The model under review builds one solid part; all positions refer to its coordinate system, in mm. A direction names the side the tool comes from. Round coordinates to 2 decimals unless told otherwise and drop trailing zeros. Write each loop counter-clockwise with the first axis right and the second up, starting at its lowest first coordinate (ties: lowest second). Pieces come first, ordered by that corner, then holes. Notation, with made-up numbers: (-12.75, -2.75) -> (33.25, -2.75) arc R24 ccw to (33.25, 16.25) -> close; hole circle Ø3 at (21.5, 21.25). An arc over 180 degrees is marked (long way). Answer as a JSON object with one key per item and string values. Group by question number.
1) To check wall thickness, follow probe 1 along X at (y, z) = (9.25, 15.75); probe 2 along Y at (x, z) = (-4.5, 16.25); probe 3 along Y at (x, z) = (-1, 19). State the ranges of each line that lie inside material, in increasing order. Write a range as [from, to].
2) We need section B-B, the plane y = 7. Write out the cut boundary in (x, z).
3) Machinability: for faces 4 (the flat face through (0, 6, -1.78)), 5 (the flat face through (-6.452, 5, 18)), 6 (the cylindrical face through (4.61, -1.38, 7.48)), 7 (the flat face through (-8.89, 5, 10)), 8 (the flat face through (8.39, -2, 9)), which of the approach directions +Z, -Z, +X, -X, +Y, -Y give a long, thin tool a straight path to every point of the face, cutting with its end or side? Answer none if there is none.
4) We need section A-A, the plane y = -0.5. Count the separate pieces of the cut face and the enclosed holes in it, then the cut area to 3 significant figures.
5) We need section D-D, the plane y = 10. Write out the cut boundary in (x, z).
6) Insertion check: pin 1 Ø6 at (x, z) = (-6.5, 20) entering from -Y; pin 2 Ø2 at (x, y) = (-1.5, 3) entering from +Z; pin 3 Ø2 at (x, z) = (3.5, 12.5) entering from -Y. Each pin has a flat end and moves straight along its axis. Give the tip position at first contact, or say it passes through.
7) Mouldability with a two-part tool opening along Z and no side actions: class faces 1 (the flat face through (0, 10.404, 18)), 2 (the cylindrical face through (-5.04, -1.38, 7.48)), 3 (the flat face through (-5, 10, 22.45)) as pulls with the +Z half, pulls with the -Z half, needs draft (parallel to the pull), parting line crosses it, or undercut.
8) We need section C-C, the plane z = 9.14. Write out the cut boundary in (x, y), then the cut area to 3 significant figures.
Autodesk Inventor part; units mm, degrees
ref_plane "YZ Plane" through (0, 0, 0) normal (1, 0, 0) x (0, 1, 0)
ref_plane "XZ Plane" through (0, 0, 0) normal (0, 1, 0) x (-1, 0, 0)
ref_plane "XY Plane" through (0, 0, 0) normal (0, 0, 1) x (1, 0, 0)
sketch "Sketch1" plane through (0, 0, 0) normal (0, 1, 0) x (-1, 0, 0)
  line L0 (8.89, 22.35) -> (-8.89, 22.35)
  line L1 (-8.89, 22.35) -> (-8.89, -1.78)
  line L2 (-8.89, -1.78) -> (8.89, -1.78)
  line L3 (8.89, -1.78) -> (8.89, 22.35)
  point P0 (0, 0)
  dimension "d0" = 24.13
  dimension "d1" = 22.35
  dimension "d2" = 17.78
  dimension "d3" = 8.89
extrude "Extrusion1" add sketch "Sketch1" along normal blind 11.25
sketch "Sketch2" plane through (-8.89, 0, 22.35) normal (0, 0, 1) x (1, 0, 0)
  line L0 (2.4376, 1.9143) -> (15.6231, 1.9143)
  line L1 (15.6231, 1.9143) -> (15.6231, 8.5296)
  line L2 (15.6231, 8.5296) -> (2.4376, 8.5296)
  line L3 (2.4376, 8.5296) -> (2.4376, 1.9143)
  line L4 (6.2307, 8.5296) -> (11.6268, 8.5296)
  line L5 (11.6268, 8.5296) -> (11.6268, 10.4036)
  line L6 (11.6268, 10.4036) -> (6.2307, 10.4036)
  line L7 (6.2307, 10.4036) -> (6.2307, 8.5296)
  point P0 (8.89, 0)
extrude "Extrusion2" cut sketch "Sketch2" against normal blind 8
sketch "Sketch3" plane through (-8.89, 0, 22.35) normal (0, 0, 1) x (1, 0, 0)
  line L0 (12.4503, 9.0228) -> (15.6135, 9.0228)
  line L1 (15.6135, 9.0228) -> (15.6135, 10.4036)
  line L2 (15.6135, 10.4036) -> (12.4503, 10.4036)
  line L3 (12.4503, 10.4036) -> (12.4503, 9.0228)
  line L4 (5.8403, 9.0228) -> (2.4376, 9.0228)
  line L5 (2.4376, 9.0228) -> (2.4376, 10.4036)
  line L6 (2.4376, 10.4036) -> (5.8403, 10.4036)
  line L7 (5.8403, 10.4036) -> (5.8403, 9.0228)
  point P0 (8.89, 0)
extrude "Extrusion3" add sketch "Sketch3" along normal blind 0.1
sketch "Sketch4" plane through (8.89, 0, 22.35) normal (1, 0, 0) x (0, 0, -1)
  line L0 (12.46, 3.4608) -> (13.96, 3.4608)
  line L1 (13.96, 3.4608) -> (13.96, -3.3)
  line L2 (13.96, -3.3) -> (12.46, -3.3)
  line L3 (12.46, -3.3) -> (12.46, 3.4608)
  line L4 (0, 0) -> (0, 11.25)
  arc A0 (12.46, -2.55) -> (13.96, -2.55) centre (13.21, -2.55) ccw
  point P0 (22.35, 0)
  dimension "d10" = 1.5
  dimension "d11" = 12.46
  dimension "d12" = 3.3
extrude "Extrusion4" add sketch "Sketch4" against normal blind 0.5 contours L0 L1 A0 L3
mirror "Mirror1" about plane through (0, 0, 0) normal (1, 0, 0) of "Extrusion4"
sketch "Sketch5" plane through (0, 0, 0) normal (0, -1, 0) x (1, 0, 0)
  circle A0 centre (-4.825, 9.14) radius 1.675
  circle A1 centre (4.825, 9.14) radius 1.675
  line L0 (-8.89, 22.35) -> (8.89, 22.35)
  point P0 (0, 0)
  dimension "d15" = 9.65
  dimension "d16" = 4.825
  dimension "d17" = 13.21
  dimension "d18" = 13.21
  dimension "d19" = 3.35
  dimension "d20" = 3.35
extrude "Extrusion5" add sketch "Sketch5" along normal blind 3.3
chamfer "Chamfer1" distance 0.5 angle 45 2 edges at (-6.5, -3.3, 9.14) (3.15, -3.3, 9.14)
sketch "Sketch6" plane through (0, 0, 0) normal (0, -1, 0) x (1, 0, 0)
  line L0 (-9.0913, 0) -> (4.8455, 0) construction
  line L1 (4.957, 2.54) -> (-8.5338, 2.54) construction
  circle A0 centre (-2.03, 0) radius 0.25
  circle A1 centre (-1.015, 2.54) radius 0.25
  line L2 (-11.1213, 0) -> (2.8155, 0) construction
  circle A2 centre (-3.045, 2.54) radius 0.25
  line L3 (-13.1513, 0) -> (0.7855, 0) construction
  circle A3 centre (-5.075, 2.54) radius 0.25
  circle A4 centre (1.015, 2.54) radius 0.25
  circle A5 centre (3.045, 2.54) radius 0.25
  circle A6 centre (5.075, 2.54) radius 0.25
  circle A7 centre (-4.06, 0) radius 0.25
  circle A8 centre (-6.09, 0) radius 0.25
  line L4 (0, 0) -> (0, 4.0434) construction
  circle A9 centre (2.03, 0) radius 0.25
  circle A10 centre (4.06, 0) radius 0.25
  circle A11 centre (6.09, 0) radius 0.25
  point P0 (-4.06, 0)
  point P1 (-6.09, 0)
  dimension "d26" = 0.5
  dimension "d27" = 0.5
  dimension "d28" = 2.54
  dimension "d29" = 1.015
  dimension "d30" = 1.015
  dimension "d33" = 2.03
  dimension "d40" = 2.03
  dimension "d47" = 2.03
extrude "Extrusion6" add sketch "Sketch6" along normal blind 3.18
sketch "Sketch7" plane through (0, 0, 0) normal (0, -1, 0) x (1, 0, 0)
  line L0 (7.52, 20.8101) -> (7.52, 18.5144) construction
  line L1 (-7.52, 21.4502) -> (-7.52, 19.3214) construction
  line L2 (-8.1276, 18.03) -> (7.9812, 18.03) construction
  line L3 (-8.0282, 15.49) -> (8.0806, 15.49) construction
  circle A0 centre (-7.52, 18.03) radius 0.25
  circle A1 centre (-7.52, 15.49) radius 0.25
  circle A2 centre (7.52, 18.03) radius 0.25
  circle A3 centre (7.52, 15.49) radius 0.25
  circle A4 centre (-7.52, 12.95) radius 0.25
  point P0 (0, 0)
  dimension "d54" = 7.52
  dimension "d55" = 15.04
  dimension "d56" = 0.5
  dimension "d57" = 0.5
  dimension "d59" = 0.5
  dimension "d60" = 0.5
  dimension "d61" = 18.03
  dimension "d63" = 2.54
  dimension "d66" = 0.5
  dimension "d67" = 2.54
extrude "Extrusion7" add sketch "Sketch7" along normal blind 3.18
properties part number "RJMG2012119A0NR_GBEConn"
Here are the results:
{
 "1": {"probe 1": "x = [-8.89, -2.66], [2.74, 8.89]", "probe 2": "y = [0, 1.91], [8.53, 11.25]", "probe 3": "y = [0, 1.91], [10.4, 11.25]"},
 "2": {"outline": "(-8.89, -1.78) -> (8.89, -1.78) -> (8.89, 22.35) -> (6.73, 22.35) -> (6.73, 14.35) -> (-6.45, 14.35) -> (-6.45, 22.35) -> (-8.89, 22.35) -> close"},
 "3": {"face 4": "-Z, +X, -X, +Y, -Y", "face 5": "+Z", "face 6": "-Y", "face 7": "+Z, -Z, -X, +Y, -Y", "face 8": "+Z, -Z, -Y"},
 "4": {"separate pieces": "21", "enclosed holes": "0", "area": "22.5 mm^2"},
 "5": {"outline": "(-8.89, -1.78) -> (8.89, -1.78) -> (8.89, 22.35) -> (6.72, 22.35) -> (6.72, 22.45) -> (3.56, 22.45) -> (3.56, 22.35) -> (2.74, 22.35) -> (2.74, 14.35) -> (-2.66, 14.35) -> (-2.66, 22.35) -> (-3.05, 22.35) -> (-3.05, 22.45) -> (-6.45, 22.45) -> (-6.45, 22.35) -> (-8.89, 22.35) -> close"},
 "6": {"pin 1": "stops at y = -3.18", "pin 2": "stops at z = 14.35", "pin 3": "stops at y = 0"},
 "7": {"face 1": "needs draft", "face 2": "undercut", "face 3": "pulls with the +Z half"},
 "8": {"outline": "(-8.89, -3.3) -> (-8.39, -3.3) -> (-8.39, 0) -> (-6.5, 0) -> (-6.5, -2.8) -> (-6, -3.3) -> (-3.65, -3.3) -> (-3.15, -2.8) -> (-3.15, 0) -> (3.15, 0) -> (3.15, -2.8) -> (3.65, -3.3) -> (6, -3.3) -> (6.5, -2.8) -> (6.5, 0) -> (8.39, 0) -> (8.39, -3.3) -> (8.89, -3.3) -> (8.89, 11.25) -> (-8.89, 11.25) -> close", "area": "225 mm^2"}
}
